from build123d import *

# Parameters (mm, degrees)
SKETCH1_W           = 10
SKETCH1_H           = 6
BOSS_EXTRUDE1_DEPTH = 9
SKETCH2_W           = 14
SKETCH2_H           = 10
BOSS_EXTRUDE2_DEPTH = 5
BOSS_EXTRUDE3_DEPTH = 7
FILLET1_R           = 2
FILLET2_R           = 1


with BuildPart() as part:
    # Sketch1 → Boss-Extrude1 (new body)
    with BuildSketch(Plane(origin=(0, 0, 0), x_dir=(1, 0, 0), z_dir=(0, 1, 0))):
        Rectangle(SKETCH1_W, SKETCH1_H)
    extrude(amount=BOSS_EXTRUDE1_DEPTH)

    # Sketch2 → Boss-Extrude2 (add)
    with BuildSketch(Plane.XZ):
        Rectangle(SKETCH2_W, SKETCH2_H)
    extrude(amount=BOSS_EXTRUDE2_DEPTH)

    # Sketch4 → Boss-Extrude3 (add, symmetric)
    with BuildSketch(Plane(origin=(0, 0, 0), x_dir=(0, 0, -1), z_dir=(1, 0, 0))):
        Polygon((-5, -5), (-32.135462652, -45), (-45.527395483, -45), (-45.527395483, -50), (-25.527395483, -50), (5, -5), align=None)
    extrude(amount=BOSS_EXTRUDE3_DEPTH, both=True)

    # Fillet1
    fillet1_edges = [part.edges().sort_by_distance(p)[0] for p in [
        (7, -2.5, -5),
        (7, -2.5, 5),
        (-7, -2.5, 5),
        (-7, -2.5, -5),
        (0, -5, -5),
        (-7, -25, 18.567731326),
        (-7, -45, 38.831429068),
        (-7, -47.5, 45.527395483),
        (0, -45, 45.527395483),
        (-7, -27.5, 10.263697742),
        (7, -25, 18.567731326),
        (7, -45, 38.831429068),
        (7, -47.5, 45.527395483),
        (7, -27.5, 10.263697742),
    ]]
    fillet(fillet1_edges, radius=FILLET1_R)

    # Fillet2
    fillet2_edges = [part.edges().sort_by_distance(p)[0] for p in [
        (-5, 9, 0),
        (0, 9, 3),
        (5, 9, 0),
        (5, 4.5, 3),
        (-5, 4.5, 3),
        (-5, 4.5, -3),
        (5, 4.5, -3),
        (0, 9, -3),
    ]]
    fillet(fillet2_edges, radius=FILLET2_R)


solid = part.part
Design review of the part built by this model. Coordinates are the model's own, in mm. A direction names the side the tool comes from. Round coordinates to 2 decimals unless told otherwise and drop trailing zeros. Write each loop counter-clockwise with the first axis right and the second up, starting at its lowest first coordinate (ties: lowest second). Pieces come first, ordered by that corner, then holes.
Item 1: Consider section D-D on x = 6. Give the boundary of the cut face in (y, z).
Item 2: For pin 1 Ø2 at (x, z) = (3.5, 4.5) entering from +Y; pin 2 Ø5 at (y, z) = (-36.5, 12.5) entering from +X; pin 3 Ø2.5 at (x, y) = (0, 3) entering from +Z; pin 4 Ø4.5 at (y, z) = (5.5, 0.5) entering from -X, all flat-tipped, find the tip position at first contact; note any pin that passes through.
Item 3: For faces 1 (the flat face through (5, 4, 0)), 2 (the cylindrical face through (-6.43, -45.6, 37.39)), 3 (the cylindrical face through (6.4, -45.57, 37.39)), 4 (the flat face through (0, 4, -3)), list the 3-axis set-ups (+Z, -Z, +X, -X, +Y, -Y) from which the entire face can be reached by the end or side of a thin tool; tool diameter is ignored.
Item 4: Consider section C-C on z = 36. Give the boundary of the cut face in (x, y).
Item 5: Consider section A-A on y = 4. Give the boundary of the cut face in (x, z), and give its area (3 significant figures).
Item 6: Wall thickness on L1, parallel to Z at x = -3.25, y = 3; L2, parallel to Z at x = 1.5, y = -3; L3, parallel to Y at x = 5, z = 36: over which ranges is each line inside the solid? List them lowest first.
Item 7: Consider section B-B on x = -2.25. Give the boundary of the cut face in (y, z), and give its area (3 significant figures).
Check values:
1. outline: (-50, 25.85) - (-5.36, -4.43) arc R1.73 ccw to (-4.39, -4.73) - (0, -4.73) - (0, 4.73) - (-5.08, 4.73) - (-45.27, 31.99) - (-45.27, 43.53) arc R1.73 ccw to (-47, 45.26) - (-50, 45.26) - close
2. pin 1: stops at y = 0
2. pin 2: passes through
2. pin 3: stops at z = 3
2. pin 4: stops at x = -5
3. face 1: +Z, -Z, +X, +Y
3. face 2: +Z, -X, +Y
3. face 3: +Z, +X, +Y
3. face 4: -Z, +X, -X, +Y
4. outline: (-7, -50) - (7, -50) - (7, -47) arc R2 ccw to (5, -45) - (-5, -45) arc R2 ccw to (-7, -47) - close
5. outline: (-5, -2) arc R1 ccw to (-4, -3) - (4, -3) arc R1 ccw to (5, -2) - (5, 2) arc R1 ccw to (4, 3) - (-4, 3) arc R1 ccw to (-5, 2) - close
5. area: 59.1 mm2
6. L1: z = -3 to 3
6. L2: z = -5 to 5
6. L3: y = -50 to -45
7. outline: (-50, 25.53) - (-5.51, -4.66) arc R2 ccw to (-4.39, -5) - (0, -5) - (0, -3) - (8, -3) arc R1 ccw to (9, -2) - (9, 2) arc R1 ccw to (8, 3) - (0, 3) - (0, 5) - (-5, 5) - (-45, 32.14) - (-45, 43.53) arc R2 ccw to (-47, 45.53) - (-50, 45.53) - close
7. area: 611 mm2
